```python
from build123d import *

# Parameters (mm, degrees)
SKETCH1_W                = 82
SKETCH1_H                = 150
BOSS_EXTRUDE1_DEPTH      = 10
SKETCH2_W                = 10
SKETCH2_H                = 45
BOSS_EXTRUDE2_DEPTH      = 82
BOSS_EXTRUDE3_DEPTH      = 42
BOSS_EXTRUDE3_DEPTH_BACK = 10
FILLET3_RADIUS           = 26
FILLET3_LENGTH           = 10
FILLET4_RADIUS           = 26
FILLET4_LENGTH           = 10
BOSS_EXTRUDE4_DEPTH      = 10
BOSS_EXTRUDE5_DEPTH      = 10
FILLET5_R                = 15
FILLET6_R                = 15
SKETCH6_R                = 8
SKETCH6_R_2              = 5.5
CUT_EXTRUDE1_DEPTH       = 131.057679512
FILLET7_R                = 3
FILLET8_R                = 3
FILLET9_R                = 3
FILLET10_R               = 3
FILLET11_R               = 2
SKETCH7_R                = 5.5
CUT_EXTRUDE2_DEPTH       = 116.043470045


with BuildPart() as part:
    # Sketch1 → Boss-Extrude1 (new body)
    with BuildSketch(Plane(origin=(0, 0, 0), x_dir=(1, 0, 0), z_dir=(0, 1, 0))):
        Rectangle(SKETCH1_W, SKETCH1_H)
    extrude(amount=BOSS_EXTRUDE1_DEPTH)

    # Sketch2 → Boss-Extrude2 (add, through all)
    with BuildSketch(Plane(origin=(41, 0, 0), x_dir=(0, 0, -1), z_dir=(1, 0, 0))):
        with Locations((70, 22.5)):
            Rectangle(SKETCH2_W, SKETCH2_H)
    extrude(amount=-BOSS_EXTRUDE2_DEPTH)

    # Sketch3 → Boss-Extrude3 (add, two sides: drawn at the far end of the back side and taken through both)
    with BuildSketch(Plane.XY.offset(-65).offset(-BOSS_EXTRUDE3_DEPTH_BACK)):
        Polygon((10, 45), (10, 10), (20, 10), (20, 45), (20, 87), (10, 87), align=None)
        Polygon((-10, 45), (-10, 87), (-20, 87), (-20, 45), (-20, 10), (-10, 10), align=None)
    extrude(amount=BOSS_EXTRUDE3_DEPTH + BOSS_EXTRUDE3_DEPTH_BACK)

    # Fillet3: full round fillet: the end face becomes a half cylinder, R = half its width
    fillet3_face = Plane((15, 87, -49), x_dir=(-1, 0, 0), z_dir=(0, 1, 0))  # on the end face: x along it, z out of the body
    fillet3_slab = fillet3_face.offset(-FILLET3_RADIUS / 2) * Box(FILLET3_LENGTH, 2 * FILLET3_RADIUS, FILLET3_RADIUS, mode=Mode.PRIVATE)  # the body's end, R deep
    fillet3_round = Plane((15, 61, -49), x_dir=(0, 1, 0), z_dir=(-1, 0, 0)) * Cylinder(FILLET3_RADIUS, FILLET3_LENGTH, mode=Mode.PRIVATE)  # its axis R under the face
    add(fillet3_slab - fillet3_round, mode=Mode.SUBTRACT)

    # Fillet4: full round fillet: the end face becomes a half cylinder, R = half its width
    fillet4_face = Plane((-15, 87, -49), x_dir=(-1, 0, 0), z_dir=(0, 1, 0))  # on the end face: x along it, z out of the body
    fillet4_slab = fillet4_face.offset(-FILLET4_RADIUS / 2) * Box(FILLET4_LENGTH, 2 * FILLET4_RADIUS, FILLET4_RADIUS, mode=Mode.PRIVATE)  # the body's end, R deep
    fillet4_round = Plane((-15, 61, -49), x_dir=(0, 1, 0), z_dir=(-1, 0, 0)) * Cylinder(FILLET4_RADIUS, FILLET4_LENGTH, mode=Mode.PRIVATE)  # its axis R under the face
    add(fillet4_slab - fillet4_round, mode=Mode.SUBTRACT)

    # Sketch4 → Boss-Extrude4 (add)
    with BuildSketch(Plane(origin=(20, 0, 0), x_dir=(0, 0, -1), z_dir=(1, 0, 0))):
        Polygon((23, 10), (23, 50), (-75, 25), (-75, 10), align=None)
    extrude(amount=-BOSS_EXTRUDE4_DEPTH)

    # Sketch5 → Boss-Extrude5 (add)
    with BuildSketch(Plane.ZY.offset(20)):
        Polygon((-23, 50), (75, 25), (75, 10), (-23, 10), align=None)
    extrude(amount=-BOSS_EXTRUDE5_DEPTH)

    # Fillet5
    fillet5_edges = [part.edges().sort_by_distance(p)[0] for p in [
        (15, 25, 75),
    ]]
    fillet(fillet5_edges, radius=FILLET5_R)

    # Fillet6
    fillet6_edges = [part.edges().sort_by_distance(p)[0] for p in [
        (-15, 25, 75),
    ]]
    fillet(fillet6_edges, radius=FILLET6_R)

    # Sketch6 → Cut-Extrude1 (cut, through all)
    with BuildSketch(Plane(origin=(20, 0, 0), x_dir=(0, 0, -1), z_dir=(1, 0, 0))):
        with Locations((49, 61)):
            Circle(SKETCH6_R)
        with Locations((-60, 17.5)):
            Circle(SKETCH6_R_2)
    extrude(amount=-CUT_EXTRUDE1_DEPTH, mode=Mode.SUBTRACT)

    # Fillet7
    fillet7_edges = [part.edges().sort_by_distance(p)[0] for p in [
        (30.5, 45, -65),
    ]]
    fillet(fillet7_edges, radius=FILLET7_R)

    # Fillet8
    fillet8_edges = [part.edges().sort_by_distance(p)[0] for p in [
        (0, 45, -65),
    ]]
    fillet(fillet8_edges, radius=FILLET8_R)

    # Fillet9
    fillet9_edges = [part.edges().sort_by_distance(p)[0] for p in [
        (-30.5, 45, -65),
    ]]
    fillet(fillet9_edges, radius=FILLET9_R)

    # Fillet10
    fillet10_edges = [part.edges().sort_by_distance(p)[0] for p in [
        (30.5, 10, -65),
        (0, 10, -65),
        (-30.5, 10, -65),
    ]]
    fillet(fillet10_edges, radius=FILLET10_R)

    # Fillet11
    fillet11_edges = [part.edges().sort_by_distance(p)[0] for p in [
        (15, 50, -23),
        (-15, 50, -23),
    ]]
    fillet(fillet11_edges, radius=FILLET11_R)

    # Sketch7 → Cut-Extrude2 (cut, through all)
    with BuildSketch(Plane(origin=(0, 10, 0), x_dir=(1, 0, 0), z_dir=(0, 1, 0))):
        with Locations(Location((31.5, 45, 0), (0, 0, 270))):
            Circle(SKETCH7_R)
        with Locations(Location((31.5, -15, 0), (0, 0, 270))):
            Circle(SKETCH7_R)
        with Locations(Location((-31.5, -15, 0), (0, 0, 90))):
            Circle(SKETCH7_R)
        with Locations(Location((-31.5, 45, 0), (0, 0, 90))):
            Circle(SKETCH7_R)
    extrude(amount=-CUT_EXTRUDE2_DEPTH, mode=Mode.SUBTRACT)


solid = part.part
```
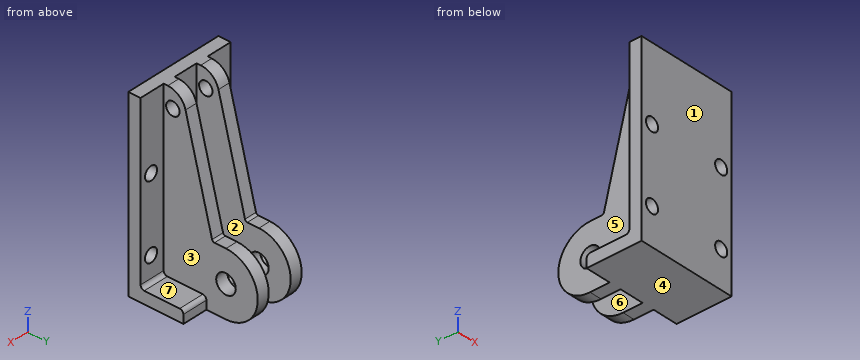
Can you work these out from the model? Positions are in its coordinate system, mm. Face numbers are marked on the shaded views. A direction names the side the tool comes from. Round coordinates to 2 decimals unless told otherwise and drop trailing zeros. Loops run counter-clockwise (first coordinate to the right, second up) from the corner with the lowest first, then second, coordinate; pieces in that order, holes last. Notation, with made-up numbers: M 48.5,-34.5 L 64.5,-34.5 A30 ccw 64.5,-7.5 Z; hole C 4,44 d8. An arc over 180 degrees is marked long. Write item = value, one per line. Start each with the question number.
(1) Suppose I cut it at A-A on x = -31.5. Write out the boundary of the cut face in (y, z), plus the area to 3 significant figures.
(2) Suppose I cut it at D-D on x = -23. Write out the boundary of the cut face in (y, z), plus the area to 3 significant figures.
(3) Suppose I cut it at C-C on z = 14.5. Write out the boundary of the cut face in (x, y).
(4) Which directions (+Z, -Z, +X, -X, +Y, -Y) give clear straight access to the entire face, cutting with the end or side of a thin tool? Please do the marked faces 4, 5, 6 and 7.
(5) Suppose I cut it at B-B on y = 58. Write out the boundary of the cut face in (x, z), plus the area to 3 significant figures.
(6) I need wall thicknesses on line 1 along X through (y, z) = (2.5, -45); line 2 along Y through (x, z) = (16, -49); line 3 along Z through (x, y) = (34.5, 9). Which ranges of each line are inside material? Lowest first, please.
(7) I'm going to push flat-ended pins straight in: P1, Ø2, axis at x = 10.5, z = 34.5, coming from the -Y side; P2, Ø7.5, axis at x = -12.5, y = 58, coming from the +Z side; P3, Ø5.5, axis at x = 32, z = -70, coming from the +Y side; P4, Ø1, axis at x = 13.5, z = -48, coming from the +Y side. Where does each tip first touch, or does it pass through?
(8) If we mould it in two halves opening along X, with no side actions, what happens to the marked faces 1, 2 and 3? For each: released by +X, released by -X, zero draft, split by the parting line, or undercut.
Answer block:
q1.outline = M 0,-75 L 45,-75 L 45,-68 A3 ccw 42,-65 L 13,-65 A3 cw 10,-62 L 10,-50.5 L 0,-50.5 Z; M 0,-39.5 L 10,-39.5 L 10,9.5 L 0,9.5 Z; M 0,20.5 L 10,20.5 L 10,75 L 0,75 Z
q1.area = 1,630 mm²
q2.outline = M 0,-75 L 45,-75 L 45,-68 A3 ccw 42,-65 L 13,-65 A3 cw 10,-62 L 10,75 L 0,75 Z
q2.area = 1,850 mm²
q3.outline = M -41,0 L -36.98,0 L -36.98,10 L -41,10 Z; M -26.02,0 L 26.02,0 L 26.02,10 L 20,10 L 20,40.43 L 10,40.43 L 10,10 L -10,10 L -10,40.43 L -20,40.43 L -20,10 L -26.02,10 Z; M 36.98,0 L 41,0 L 41,10 L 36.98,10 Z
q4.face_4 = -Z, +X, -X, +Y, -Y
q4.face_5 = +Z, -X, +Y
q4.face_6 = +Z, +Y
q4.face_7 = +Z, +X, +Y
q5.outline = M -20,-75 L -10,-75 L -10,-56.42 L -20,-56.42 Z; M -20,-41.58 L -10,-41.58 L -10,-23 L -20,-23 Z; M 10,-75 L 20,-75 L 20,-56.42 L 10,-56.42 Z; M 10,-41.58 L 20,-41.58 L 20,-23 L 10,-23 Z
q5.area = 743 mm²
q6.line_1 = -41 to -37, -26 to 26, 37 to 41
q6.line_2 = 0 to 53, 69 to 87
q6.line_3 = -75 to -49.61, -40.39 to 10.39, 19.61 to 75
q7.P1 = 0
q7.P2 = -23
q7.P3 = 45
q7.P4 = 87
q8.face_1 = zero draft
q8.face_2 = undercut
q8.face_3 = released by +X
